from build123d import *

# Parameters (mm, degrees)
RESSALTO_EXTRUS_O1_DEPTH = 25
RESSALTO_EXTRUS_O2_DEPTH = 4
RESSALTO_EXTRUS_O4_DEPTH = 4
PADR_O_LINEAR1_COUNT     = 2
PADR_O_LINEAR1_PITCH     = 11
CORTE_EXTRUS_O1_DEPTH    = 7
ESBO_O6_R                = 2
CORTE_EXTRUS_O2_DEPTH    = 5
CORTE_EXTRUS_O3_DEPTH    = 5
FILETE2_R                = 2
FILETE3_R                = 2
FILETE4_R                = 2
FILETE5_R                = 2
FILETE6_R                = 2


with BuildPart() as part:
    # Esboço1 → Ressalto-extrusão1 (new body)
    with BuildSketch(Plane.XY):
        Polygon((0, 0), (-15, 0), (-15, 15), (-11, 15), (-11, 4), (0, 4), align=None)
    extrude(amount=RESSALTO_EXTRUS_O1_DEPTH)

    # Esboço2 → Ressalto-extrusão2 (add)
    with BuildSketch(Plane(origin=(0, 0, 0), x_dir=(-1, 0, 0), z_dir=(0, 0, -1))):
        with BuildLine():
            Line((0, 4), (11, 4))
            Line((11, 4), (11, 15))
            ThreePointArc((11, 15), (7.778174593, 7.221825407), (0, 4))
        make_face()
    extrude(amount=-RESSALTO_EXTRUS_O2_DEPTH)

    # Esboço3 → Ressalto-extrusão4 (add)
    with BuildSketch(Plane(origin=(0, 0, 0), x_dir=(0, 0, -1), z_dir=(1, 0, 0))):
        Polygon((0, 0), (-4, 0), (-4, -2), (-2, -2), align=None)
    ressalto_extrus_o4 = extrude(amount=-RESSALTO_EXTRUS_O4_DEPTH)

    # Padrão linear1: Ressalto-extrusão4 ×2
    with Locations(*[(-i * PADR_O_LINEAR1_PITCH, 0, 0) for i in range(1, PADR_O_LINEAR1_COUNT)]):
        add(ressalto_extrus_o4)

    # Esboço5 → Corte-extrusão1 (cut, through all)
    with BuildSketch(Plane(origin=(0, 4, 0), x_dir=(1, 0, 0), z_dir=(0, 1, 0))):
        with BuildLine():
            Line((-7.25, -20), (-7.25, -16))
            ThreePointArc((-7.25, -16), (-5.5, -14.25), (-3.75, -16))
            Line((-3.75, -16), (-3.75, -20))
            ThreePointArc((-3.75, -20), (-5.5, -21.75), (-7.25, -20))
        make_face()
    extrude(amount=-CORTE_EXTRUS_O1_DEPTH, mode=Mode.SUBTRACT)

    # Esboço6 → Corte-extrusão2 (cut, through all)
    with BuildSketch(Plane(origin=(-11, 0, 0), x_dir=(0, 0, -1), z_dir=(1, 0, 0))):
        with Locations((-9, 9.5)):
            Circle(ESBO_O6_R)
    extrude(amount=-CORTE_EXTRUS_O2_DEPTH, mode=Mode.SUBTRACT)

    # Esboço8 → Corte-extrusão3 (cut, through all)
    with BuildSketch(Plane(origin=(-11, 0, 0), x_dir=(0, 0, -1), z_dir=(1, 0, 0))):
        with BuildLine():
            Line((-25, 4), (-25, 15))
            Line((-25, 15), (-14, 15))
            ThreePointArc((-14, 15), (-17.221825407, 7.221825407), (-25, 4))
        make_face()
    extrude(amount=-CORTE_EXTRUS_O3_DEPTH, mode=Mode.SUBTRACT)

    # Filete2
    filete2_edges = [part.edges().sort_by_distance(p)[0] for p in [
        (-13, 15, 14),
    ]]
    fillet(filete2_edges, radius=FILETE2_R)

    # Filete3
    filete3_edges = [part.edges().sort_by_distance(p)[0] for p in [
        (0, 2, 25),
    ]]
    fillet(filete3_edges, radius=FILETE3_R)

    # Filete4
    filete4_edges = [part.edges().sort_by_distance(p)[0] for p in [
        (-15, 2, 25),
    ]]
    fillet(filete4_edges, radius=FILETE4_R)

    # Filete5
    filete5_edges = [part.edges().sort_by_distance(p)[0] for p in [
        (0, 2, 0),
    ]]
    fillet(filete5_edges, radius=FILETE5_R)

    # Filete6
    filete6_edges = [part.edges().sort_by_distance(p)[0] for p in [
        (-13, 15, 0),
    ]]
    fillet(filete6_edges, radius=FILETE6_R)


solid = part.part
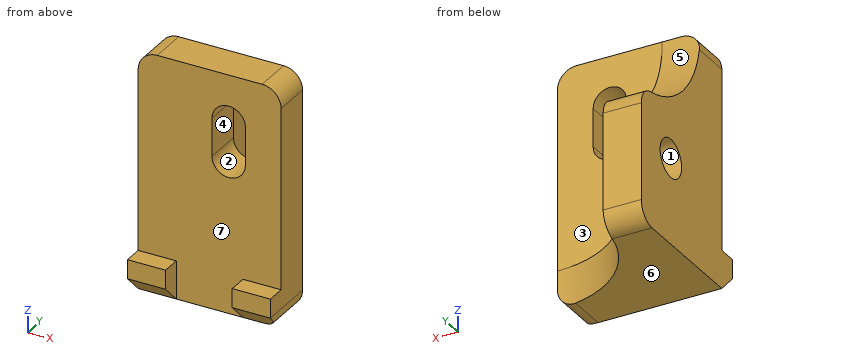
The listing builds one solid part. Answer for the finished solid, in the listing's coordinates (mm). Face numbers are marked on the shaded views. A direction names the side the tool comes from. Coordinates: 2 decimals unless noted, no trailing zeros. Order: outer loops, then holes, each group sorted by start corner. A loop starts at its lowest first (then second) coordinate and runs counter-clockwise, first axis right, second up.
Q1. Which of the six approach directions +Z, -Z, +X, -X, +Y, -Y give full straight-line access (tool end or side, diameter ignored) to the marked faces 1, 2 and 3?
Q2. A cutting plane is placed at D-D, the plane y = 6.5. Write down the section's boundary in (x, z).
Q3. A cutting plane is placed at A-A, the plane z = 9. Write down the section's boundary in (x, y).
Q4. A cutting plane is placed at C-C, the plane y = 2.5. Write down the section's boundary in (x, z).
Q5. A cutting plane is placed at B-B, the plane x = -6.75. Write down the section's boundary in (y, z).
Q6. Given P1, Ø9, axis at x = -6, y = 11, coming from the +Z side; P2, Ø2, axis at y = -1, z = 1.5, coming from the +X side; P3, Ø4, axis at y = 11.5, z = 16, coming from the +X side; P4, Ø1, axis at x = -4, z = 16, coming from the -Y side, each flat-ended and moving along its own axis, determine where each tip first touches the part or whether it passes through.
Q7. Consider line 1 (Y direction, x = -14, z = 9); line 2 (Y direction, x = -4.5, z = 8.25); line 3 (X direction, y = 11.5, z = 6.75). Determine where each line is inside the solid, lowest interval first.
Q8. For a pull along Z with two mould halves and no side action, classify the marked faces 4, 5, 6 and 7 as pulls with the +Z half, pulls with the -Z half, needs draft (parallel to the pull), parting line crosses it, or undercut.
Answers follow:
1. face 1: +X, -X
1. face 2: +Y, -Y
1. face 3: +Z, +X, +Y
2. outline: (-15, 0) - (-6.98, 0) - (-6.98, 4) - (-11, 4) - (-11, 18.02) - (-15, 18.02) - close
3. outline: (-15, 0) - (0, 0) - (0, 4) - (-11, 4) - (-11, 7.5) - (-15, 7.5) - close; (-15, 11.5) - (-11, 11.5) - (-11, 15) - (-15, 15) - close
4. outline: (-15, 0) - (-2, 0) arc R2 ccw to (0, 2) - (0, 23) arc R2 ccw to (-2, 25) - (-13, 25) arc R2 ccw to (-15, 23) - close; hole (-7.25, 16) arc R1.75 ccw to (-3.75, 16) - (-3.75, 20) arc R1.75 ccw to (-7.25, 20) - close
5. outline: (0, 0) - (6.31, 0) - (6.31, 4) - (4, 4) - (4, 14.78) - (0, 14.78) - close; (0, 21.22) - (4, 21.22) - (4, 25) - (0, 25) - close
6. P1: stops at z = 4
6. P2: stops at x = 0
6. P3: stops at x = -11
6. P4: stops at y = 0
7. line 1: y = 0 to 7.5, 11.5 to 15
7. line 2: y = 0 to 4
7. line 3: x = -15 to -11
8. face 4: undercut
8. face 5: pulls with the +Z half
8. face 6: pulls with the -Z half
8. face 7: needs draft
